Study the drawing (mm; zero at the part's minimum x, y, z) and answer. Coordinates: 2 decimals unless noted, no trailing zeros. Loops run counter-clockwise (first coordinate to the right, second up) from the corner with the lowest first, then second, coordinate; pieces in that order, holes last.
Q1. Section A-A (z = 12) is taken. Give the vertices of the cut face in (x, y).
Q2. Section C-C (y = 10) is taken. Give the vertices of the cut face in (x, z), then the cut area to 3 significant figures.
Q3. Section B-B (x = 15.75) is taken. Give the vertices of the cut face in (y, z).
Q4. Straight lines are drawn through the part: line 1 (Z direction, x = 11.75, y = 23); line 2 (Z direction, x = 7.5, y = 13.5); line 3 (Z direction, x = 5, y = 2). For each, find the intervals that lie inside material, in ascending order.
Q5. The mould has two halves that part along X. Classify the marked faces 1, 2, 3 and 4: pulls with the +X half, pulls with the -X half, needs draft (parallel to the pull), parting line crosses it, or undercut.
Q6. Flat-ended cylindrical pins translate along their axes: P1, Ø3.5, axis at y = 23, z = 12, coming from the +X side; P2, Ø2, axis at y = 10, z = 25, coming from the +X side. Find the tip coordinate at first contact, or state that the pin passes through.
Q7. Section D-D (z = 4) is taken. Give the vertices of the cut face in (x, y).
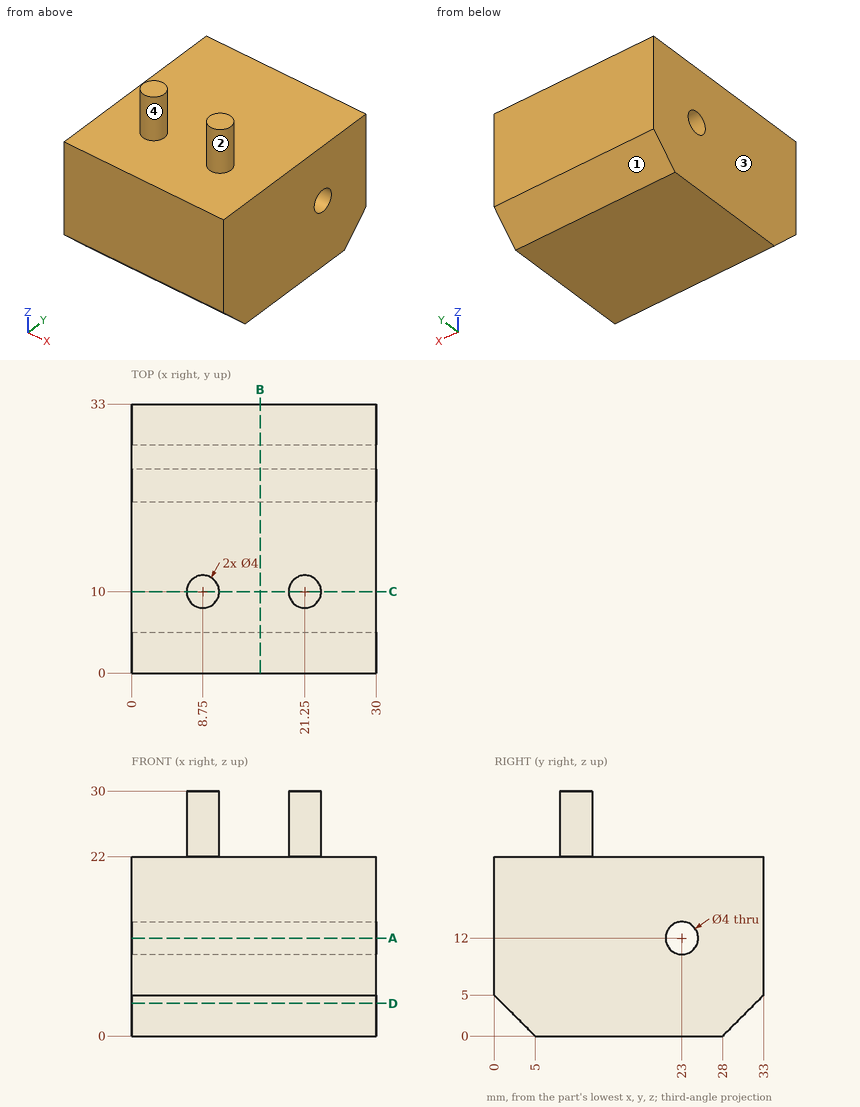
Numbers:
1. outline: (0, 0) - (30, 0) - (30, 21) - (0, 21) - close; (0, 25) - (30, 25) - (30, 33) - (0, 33) - close
2. outline: (0, 0) - (30, 0) - (30, 22) - (23.25, 22) - (23.25, 30) - (19.25, 30) - (19.25, 22) - (10.75, 22) - (10.75, 30) - (6.75, 30) - (6.75, 22) - (0, 22) - close
2. area: 724 mm2
3. outline: (0, 5) - (5, 0) - (28, 0) - (33, 5) - (33, 22) - (0, 22) - close; hole circle Ø4 at (23, 12)
4. line 1: z = 0 to 10, 14 to 22
4. line 2: z = 0 to 22
4. line 3: z = 3 to 22
5. face 1: needs draft
5. face 2: undercut
5. face 3: pulls with the -X half
5. face 4: undercut
6. P1: passes through
6. P2: stops at x = 23.25
7. outline: (0, 1) - (30, 1) - (30, 32) - (0, 32) - close
